Autodesk Inventor part; units mm, degrees
ref_plane "Płaszczyzna konstrukcyjna1" through (0, 2, 0) normal (0, 1, 0) x (1, 0, 0)
ref_plane "YZ Plane" through (0, 0, 0) normal (1, 0, 0) x (0, 1, 0)
ref_plane "XZ Plane" through (0, 0, 0) normal (0, 1, 0) x (-1, 0, 0)
sketch "Szkic1" plane through (0, 0, 0) normal (0, 1, 0) x (-1, 0, 0)
  circle A0 centre (0, 22.5) radius 2
  circle A1 centre (0, -22.5) radius 2
  circle A2 centre (0, 22.5) radius 11.25 construction
  circle A3 centre (0, -22.5) radius 11.25 construction
  circle A4 centre (0, 0) radius 11.25
  circle A5 centre (-15.3043, -4.6667) radius 4.75 construction
  circle A6 centre (-15.3043, -4.6667) radius 12.25 construction
  circle A7 centre (-18.2464, 15.6211) radius 8.25 construction
  circle A8 centre (-18.2464, 15.6211) radius 1
  circle A9 centre (-15.3043, -4.6667) radius 1.5
  line L0 (17, 55) -> (-27.5543, 55)
  line L1 (-27.5543, 55) -> (-27.5543, -55)
  line L2 (-27.5543, -55) -> (17, -55)
  line L3 (17, -55) -> (17, 55)
  circle A10 centre (0, 22.5) radius 17 construction
  circle A11 centre (0, -22.5) radius 17 construction
  circle A12 centre (0, 0) radius 14.5 construction
  line L4 (12.5, 7.3485) -> (12.5, -7.3485) construction
  line L5 (-12.5, 7.3485) -> (-12.5, -7.3485) construction
  circle A13 centre (12.0332, -7.1556) radius 8.25 construction
  circle A14 centre (12.0332, -7.1556) radius 2.75 construction
  circle A15 centre (14.255, 9.1942) radius 8.25 construction
  circle A16 centre (14.255, 9.1942) radius 1
  circle A17 centre (12.0332, -7.1556) radius 1
  circle A18 centre (-3.8336, 8) radius 8.25 construction
  circle A19 centre (-3.8336, 8) radius 1
  circle A20 centre (-3.8336, 8) radius 2.75 construction
  circle A21 centre (4.6517, 1) radius 8.25 construction
  circle A22 centre (4.6517, 1) radius 1
  circle A23 centre (4.6517, 1) radius 2.75 construction
  line L6 (-27.5543, -0.6454) -> (-7, -30)
  line L7 (-7, -30) -> (-7, -64)
  line L8 (-7, -64) -> (5, -64)
  line L9 (5, -64) -> (5, -30)
  line L10 (5, -30) -> (17, -12.8622)
  line L11 (17, 12.5) -> (2, 27.5)
  line L12 (2, 27.5) -> (-12.5543, 27.5)
  line L13 (-12.5543, 27.5) -> (-27.5543, 12.5)
  circle A24 centre (0, 0) radius 2
  circle A25 centre (-9.3126, 0) radius 11.25 construction
  circle A26 centre (-9.3126, 0) radius 2
  circle A27 centre (-15.3227, 0) radius 11.25 construction
  circle A28 centre (-15.3227, 0) radius 2
  point P0 (-7, -55)
  point P1 (5, -55)
  dimension "d0" = 4
  dimension "d1" = 4
  dimension "d2" = 22.5
  dimension "d3" = 22.5
  dimension "d4" = 22.5
  dimension "d5" = 22.5
  dimension "d6" = 22.5
  dimension "d7" = 9.5
  dimension "d8" = 24.5
  dimension "d9" = 16.5
  dimension "d10" = 2
  dimension "d11" = 3
  dimension "d12" = 34
  dimension "d13" = 34
  dimension "d14" = 29
  dimension "d15" = 25
  dimension "d16" = 17
  dimension "d17" = 55
  dimension "d18" = 110
  dimension "d21" = 16.5
  dimension "d22" = 5.5
  dimension "d23" = 16.5
  dimension "d24" = 45
  dimension "d26" = 2
  dimension "d27" = 2
  dimension "d28" = 16.5
  dimension "d29" = 2
  dimension "d30" = 5.5
  dimension "d33" = 16.5
  dimension "d34" = 27.5543
  dimension "d35" = 2
  dimension "d36" = 5.5
  dimension "d39" = 12
  dimension "d40" = 12
  dimension "d41" = 0
  dimension "d42" = 9
  dimension "d43" = 145
  dimension "d44" = 145
  dimension "d45" = 25
  dimension "d46" = 45
  dimension "d47" = 45
  dimension "d48" = 15
  dimension "d49" = 5
  dimension "d50" = 0
  dimension "d63" = 1
  dimension "d64" = 8
  dimension "d65" = 4
  dimension "d66" = 22.5
  dimension "d67" = 0
  dimension "d68" = 4
  dimension "d69" = 22.5
  dimension "d70" = 0
  dimension "d71" = 4
ref_plane "Płaszczyzna konstrukcyjna1" through (0, 2, 0) normal (0, 1, 0) x (1, 0, 0)
sketch "Szkic2" plane through (0, 2, 0) normal (0, 1, 0) x (1, 0, 0)
  circle A0 centre (0, -22.5) radius 2
  circle A1 centre (-14.255, -9.1942) radius 1
  circle A2 centre (3.8336, -8) radius 1
  circle A3 centre (-4.6517, -1) radius 1
  circle A4 centre (15.3043, 4.6667) radius 1.5
  circle A5 centre (0, 22.5) radius 2
  circle A6 centre (-12.0332, 7.1556) radius 1
  circle A7 centre (18.2464, -15.6211) radius 1
  circle A8 centre (0, -22.5) radius 2
  circle A9 centre (-14.255, -9.1942) radius 1
  circle A10 centre (3.8336, -8) radius 1
  circle A11 centre (-4.6517, -1) radius 1
  circle A12 centre (15.3043, 4.6667) radius 1.5
  circle A13 centre (18.2464, -15.6211) radius 1
  circle A14 centre (0, 22.5) radius 2
  circle A15 centre (-12.0332, 7.1556) radius 1
  circle A16 centre (0, -22.5) radius 3
  circle A17 centre (-14.255, -9.1942) radius 2
  circle A18 centre (3.8336, -8) radius 2
  circle A19 centre (-4.6517, -1) radius 2
  circle A20 centre (18.2464, -15.6211) radius 2
  circle A21 centre (15.3043, 4.6667) radius 2.5
  circle A22 centre (0, 22.5) radius 3
  circle A23 centre (-12.0332, 7.1556) radius 2
  point P0 (0, 0)
  dimension "d53" = 1
  dimension "d54" = 1
  dimension "d55" = 1
  dimension "d56" = 1
  dimension "d57" = 1
  dimension "d58" = 1
  dimension "d59" = 1
  dimension "d60" = 1
extrude "Wyciągnięcie proste6" add sketch "Szkic1" along normal blind 2 contours A4 A26 | L3 L10 L9 L2 L7 L6 L1 L13 L12 L11 picked at (-5.8126, -3.4695)
extrude "Wyciągnięcie proste7" add sketch "Szkic2" along normal blind 2
The listing builds one solid part. Answer for the finished solid, in the listing's coordinates (mm). A direction names the side the tool comes from. Coordinates: 2 decimals unless noted, no trailing zeros. Write each loop counter-clockwise with the first axis right and the second up, starting at its lowest first coordinate (ties: lowest second). Pieces come first, ordered by that corner, then holes. Notation, with made-up numbers: (82, 8.25) -> (104, 8.25) arc R8 cw to (104, 22.25) -> close; hole circle Ø10 at (29.5, -14.75). An arc over 180 degrees is marked (long way). Write each question's results on one line, items separated by ' | '. Start each with the question number.
1) A cutting plane is placed at D-D (x = 9.5). Determine the outline of the cut face in (y, z).
2) A cutting plane is placed at B-B (y = 1.15). Count the separate pieces of the cut face and the enclosed holes in it, then the cut area to 3 significant figures.
3) A cutting plane is placed at C-C (z = -39). Determine the outline of the cut face in (x, y).
4) A tool of negligible diameter and unlimited length cuts with its end or side. For faces 4 (the flat face through (3, 4, 7)), 5 (the cylindrical face through (12.807, 2.986, -4.557)), from which of +Z, -Z, +X, -X, +Y, -Y can it reach the whole face along a straight path? Write none if from no direction.
5) Flat-ended cylindrical pins translate along their axes: pin 1 Ø0.6 at (y, z) = (1, -45.5) entering from -X; pin 2 Ø0.6 at (y, z) = (1, -46.5) entering from +X; pin 3 Ø2.5 at (x, z) = (3.83, 8) entering from +Y; pin 4 Ø8 at (x, z) = (-8, -39) entering from +Y. Find the tip coordinate at first contact, or state that the pin passes through.
6) Straight lines are drawn through the part: probe 1 along Z at (x, y) = (-0.5, 3.7); probe 2 along Z at (x, y) = (15, 0.85); probe 3 along X at (y, z) = (1.15, 8). For each, find the intervals that lie inside material, in ascending order.
7) For a pull along Z with two mould halves and no side action, classify faces 1 (the cylindrical face through (-13.6, 3, -8.4)), 2 (the flat face through (-10.916, 0.986, -21.551)), 3 (the flat face through (1, 0, -4)) as +Z half, -Z half, draft (parallel to the pull), parting line (faces both ways), or undercut.
Values follow:
1) outline: (0, -26.43) -> (2, -26.43) -> (2, -1.99) -> (0, -1.99) -> close; (0, 1.99) -> (2, 1.99) -> (2, 27.5) -> (0, 27.5) -> close
2) separate pieces: 1 | enclosed holes: 11 | area: 2,150 mm²
3) outline: (-5, 0) -> (7, 0) -> (7, 2) -> (-5, 2) -> close
4) face 4: +Z, -Z, +X, -X, +Y | face 5: +Y
5) pin 1: x = -5 | pin 2: x = 7 | pin 3: y = 4 | pin 4: y = 2
6) probe 1: -25.46 to -24.44, -20.56 to -19.54, 19.54 to 20.56, 24.44 to 25.46 | probe 2: -18.57 to -6.14, -3.2 to -1.97, 1.97 to 25.05 | probe 3: -17 to 2.83, 4.83 to 27.55
7) face 1: undercut | face 2: -Z half | face 3: draft
